from build123d import *


with BuildPart() as f1:
    # F0 (on Front) → F1 (revolve)
    with BuildSketch(Plane.XZ):
        with BuildLine():
            Line((-3, 7.5), (-3, 0))
            Line((-3, 0), (-2.5, 0))
            Line((-2.5, 0), (-2.5, 7.5))
            Line((-2.5, 7.5), (0, 7.5))
            Line((0, 7.5), (0, 8.867949))
            ThreePointArc((0, 8.867949), (-3.588595, 9.269139), (-7, 10.452899))
            Line((-7, 10.452899), (-8.5, 10.452899))
            Line((-8.5, 10.452899), (-8.5, 7.5))
            Line((-8.5, 7.5), (-3, 7.5))
        make_face()
    revolve(axis=Axis((0, 0, 8.183975), (0, 0, -1)))


solid = f1.part
Here's how the part is built. I have some questions about the finished solid (model axes, mm). A direction names the side the tool comes from. Coordinates: 2 decimals unless noted, no trailing zeros. Write each loop counter-clockwise with the first axis right and the second up, starting at its lowest first coordinate (ties: lowest second). Pieces come first, ordered by that corner, then holes.
1) If we section it at B-B (z = 8.25): List the corners of the cut face in (x, y) for me.
Filled in:
outline: circle Ø17 at (0, 0)
2) If I drill on line 1 (Y direction, x = 0, z = 2.25); line 2 (Z direction, x = -6.5, y = -5.25); line 3 (Y direction, x = -1, z = 4.75), over which ranges is the centre line in solid material (lowest first)?
Filled in:
line 1: y = -3 to -2.5, 2.5 to 3
line 2: z = 7.5 to 10.45
line 3: y = -2.83 to -2.29, 2.29 to 2.83
3) Which directions (+Z, -Z, +X, -X, +Y, -Y) give clear straight access to the entire face, cutting with the end or side of a thin tool? Please do faces 5 (the face through (-4.57, 7.167, 8.956)), 6 (the face through (-4, 0, 7.5)).
Filled in:
face 5: +Z, -Z
face 6: -Z
4) I'm going to push flat-ended pins straight in: pin 1 (6 mm diameter, centred on y = 0, z = 2.5, fed in from +X); pin 2 (4 mm diameter, centred on x = -6, y = 6.5, fed in from -Z); pin 3 (3 mm diameter, centred on x = -6.5, z = 9, fed in from +Y). Where does each tip first touch, or does it pass through?
Filled in:
pin 1: stops at x = 3
pin 2: stops at z = 7.5
pin 3: stops at y = 6.87
5) Thinking about a two-plate mould opening in Y: for faces 1 (the face through (0, 0, 7.5)), 2 (the face through (3, 0, 4)), 3 (the face through (0.54, -2.44, 3.8)), 4 (the face through (2, 2, 0)), which applies, +Y half, -Y half, draft (parallel to the pull), parting line (faces both ways), or undercut?
Filled in:
face 1: undercut
face 2: parting line
face 3: undercut
face 4: draft
6) If we section it at A-A (z = 2.75): List the corners of the cut face in (x, y) for me, plus the area to 3 significant figures.
Filled in:
outline: circle Ø6 at (0, 0); hole circle Ø5 at (0, 0)
area: 8.64 mm2
